from build123d import *

# Parameters (mm, degrees)
F0_W     = 50.8
F0_H     = 101.6
F1_DEPTH = 50.8
F2_W     = 50.8
F2_H     = 25.4
F3_DEPTH = 50.8
F5_DEPTH = 152.4
F6_W     = 152.4
F6_H     = 50.8
F7_DEPTH = 25.4


with BuildPart() as f1:
    # F0 (on Top) → F1 (new body)
    with BuildSketch(Plane.XY):
        with Locations((-106.38359, 33.388032)):
            Rectangle(F0_W, F0_H)
    extrude(amount=F1_DEPTH)

    # F2 (on face) → F3 (join)
    with BuildSketch(Plane.XY.offset(50.8)):
        with Locations((-106.38359, 71.488032)):
            Rectangle(F2_W, F2_H)
    extrude(amount=F3_DEPTH)

    # F4 (on face) → F5 (join)
    with BuildSketch(Plane.YZ.offset(-80.98359)):
        Polygon((58.788032, 50.8), (7.988032, 50.8), (7.988032, 0), (84.188032, 0), (84.188032, 101.6), (58.788032, 101.6), align=None)
    extrude(amount=F5_DEPTH)

    # F6 (on face) → F7 (cut)
    with BuildSketch(Plane.XZ.offset(-58.788032)):
        with Locations((-4.78359, 76.2)):
            Rectangle(F6_W, F6_H)
    extrude(amount=-F7_DEPTH, mode=Mode.SUBTRACT)


solid = f1.part
Geometry: final body of the model. Coordinates: model frame, mm. A direction names the side the tool comes from. Give positions to 0.01 mm unless a question says otherwise; leave off trailing zeros. Loops run counter-clockwise (first coordinate to the right, second up) from the corner with the lowest first, then second, coordinate; pieces in that order, holes last. Notation, with made-up numbers: (3.25, -5.75) - (58.25, -5.75) arc R34 cw to (58.25, 28.25) - close; hole circle Ø10 at (79.25, 15.25). An arc over 180 degrees is marked (long way). One line per question, with ' | ' between items. Start each with the question number.
(1) Section query C-C on x = 14.5. Return loops of the section in (y, z).
(2) Section query D-D on y = -0.5. Return loops of the section in (x, z).
(3) Section query A-A on z = 23. Return loops of the section in (x, y).
(4) Ray query, line 1 (Y direction, x = -39.5, z = 9); line 2 (Y direction, x = -123, z = 91); line 3 (X direction, y = 1, z = 21.5). Return the intervals inside material, ascending. Write a range as from..to.
(5) Section query B-B on y = 77. Return loops of the section in (x, z).
(6) Reachability of faces 1 (the flat face through (-80.984, -5, 25)), 2 (the flat face through (-107, 58.788, 77)), 3 (the flat face through (-80.984, 71, 76)) from +Z, -Z, +X, -X, +Y, -Y: full face, straight path, thin tool, end or side. Return the list, or none.
(7) Contact query for flat-ended pins moving along their axis: pin 1 (4 mm diameter, centred on x = 7, y = 69.5, fed in from +Z); pin 2 (12.5 mm diameter, centred on y = 73.5, z = 80, fed in from +X). Output: stop coordinate, or through.
The answers:
1) outline: (7.99, 0) - (84.19, 0) - (84.19, 50.8) - (7.99, 50.8) - close
2) outline: (-131.78, 0) - (-80.98, 0) - (-80.98, 50.8) - (-131.78, 50.8) - close
3) outline: (-131.78, -17.41) - (-80.98, -17.41) - (-80.98, 7.99) - (71.42, 7.99) - (71.42, 84.19) - (-131.78, 84.19) - close
4) line 1: 7.99..84.19 | line 2: 58.79..84.19 | line 3: -131.78..-80.98
5) outline: (-131.78, 0) - (71.42, 0) - (71.42, 50.8) - (-80.98, 50.8) - (-80.98, 101.6) - (-131.78, 101.6) - close
6) face 1: +Z, -Z, +X, -Y | face 2: +Z, +X, -X, -Y | face 3: +Z, +X, +Y, -Y
7) pin 1: z = 50.8 | pin 2: x = -80.98
